Part model, mm, in its own coordinate system. A direction names the side the tool comes from. Round coordinates to 2 decimals unless told otherwise and drop trailing zeros. Write each loop counter-clockwise with the first axis right and the second up, starting at its lowest first coordinate (ties: lowest second). Pieces come first, ordered by that corner, then holes. Notation, with made-up numbers: M -37.5,41 L 12.5,41 A6 cw 12.5,51 Z; hole C 34.25,37.5 d3. An arc over 180 degrees is marked long. Use one line per item in the form item = value. Start each with the question number.
Item 1: Probe L1, parallel to Z at x = -18, y = 173; L2, parallel to Z at x = -14, y = 80.5; L3, parallel to Y at x = -21.5, z = 3.5. List the from-to ranges inside material, lowest first.
Item 2: Cut at B-B, the plane y = 94. Give the cut face in (x, z), then the cut area to 3 significant figures.
Item 3: Cut at A-A, the plane z = 3. Give the cut face in (x, y), then the cut area to 3 significant figures.
Item 4: Flat gauge pins, fed straight in: pin 1 Ø0.8 at (y, z) = (117.5, 6.5) entering from +X; pin 2 Ø3.5 at (x, z) = (-8.5, 2) entering from -Y; pin 3 Ø7.5 at (x, y) = (-4, 57) entering from +Z. Where does each tip first touch, or does it go through?
Item 5: Which spindle directions (+Z, -Z, +X, -X, +Y, -Y) get a long thin tool onto all of the face, cutting with end or side? Do faces 4 (the face through (-13, 89, 6)), 5 (the face through (-10, 89, 0)), 6 (the face through (-16.5, 174.58, 3.07)). Say none if no direction does.
Item 6: Mould opens along Z. For faces 1 (the face through (-22.9, 88.74, 3.55)), 2 (the face through (-19.5, -4.93, 2.93)), 3 (the face through (-15, 89, 3)) say: +Z half, -Z half, draft (parallel to the pull), parting line (faces both ways), or undercut.
Item 7: Cut at C-C, the plane x = -26.5. Give the cut face in (y, z).
Autodesk Fusion 360 part; units mm, degrees
sketch "Sketch1" plane through (0, 0, 0) normal (0, 1, 0) x (1, 0, 0)
  line L0 (-30, 0) -> (10, 0)
  line L1 (10, 0) -> (10, -1)
  line L2 (10, -1) -> (-15, -1)
  line L3 (-15, -1) -> (-15, -6)
  line L4 (-15, -6) -> (-10, -6)
  line L5 (-10, -6) -> (-10, -7)
  line L6 (-10, -7) -> (-16, -7)
  line L7 (-16, -7) -> (-30, 0)
  dimension "d1" = 40
  dimension "d2" = 1
sketch "Sketch2" plane through (0, 0, 0) normal (0, 1, 0) x (1, 0, 0)
extrude "Extrude1" add sketch "Sketch1" along normal blind 200
sketch "Sketch3" plane through (0, 0, 0) normal (0, -1, 0) x (1, 0, 0)
  line L0 (-10, 7) -> (-16, 7)
  line L1 (-16, 7) -> (-30, 0)
  line L2 (-30, 0) -> (10, 0)
  line L3 (10, 0) -> (10, 1)
  line L4 (10, 1) -> (-15, 1)
  line L5 (-15, 1) -> (-15, 6)
  line L6 (-15, 6) -> (-10, 6)
  line L7 (-10, 6) -> (-10, 7)
  circle A0 centre (-18, 3) radius 1.5
  dimension "d5" = 3
  dimension "d6" = 3
  dimension "d7" = 3
extrude "Extrude2" add sketch "Sketch3" along normal blind 10 contours A0
sketch "Sketch4" plane through (0, 0, 0) normal (0, 1, 0) x (1, 0, 0)
sketch "Sketch5" plane through (0, 200, 0) normal (0, 1, 0) x (-1, 0, 0)
  line L0 (16, 7) -> (10, 7)
  line L1 (10, 7) -> (10, 6)
  line L2 (10, 6) -> (15, 6)
  line L3 (15, 6) -> (15, 1)
  line L4 (15, 1) -> (-10, 1)
  line L5 (-10, 1) -> (-10, 0)
  line L6 (-10, 0) -> (30, 0)
  line L7 (30, 0) -> (16, 7)
  circle A0 centre (18, 3) radius 1.5
  dimension "d10" = 3
  dimension "d11" = 3
  dimension "d12" = 3
extrude "Extrude3" cut sketch "Sketch5" against normal blind 11 contours A0
sketch "Sketch6" plane through (0, 200, 0) normal (0, 1, 0) x (-1, 0, 0)
  line L0 (16, 7) -> (10, 7)
  line L1 (10, 7) -> (10, 6)
  line L2 (10, 6) -> (15, 6)
  line L3 (15, 6) -> (15, 1)
  line L4 (15, 1) -> (-10, 1)
  line L5 (-10, 1) -> (-10, 0)
  line L6 (-10, 0) -> (30, 0)
  line L7 (30, 0) -> (16, 7)
extrude "Extrude4" cut sketch "Sketch6" against normal blind 20
sketch "Sketch7" plane through (0, 0, 0) normal (0, 1, 0) x (1, 0, 0)
sketch "Sketch8" plane through (0, 180, 0) normal (0, 1, 0) x (-1, 0, 0)
  line L0 (30, 0) -> (16, 7)
  line L1 (16, 7) -> (10, 7)
  line L2 (10, 7) -> (10, 6)
  line L3 (10, 6) -> (15, 6)
  line L4 (15, 6) -> (15, 1)
  line L5 (15, 1) -> (-10, 1)
  line L6 (-10, 1) -> (-10, 0)
  line L7 (-10, 0) -> (30, 0)
  circle A0 centre (18, 3) radius 1.5
  dimension "d17" = 3
  dimension "d18" = 3
  dimension "d19" = 3
extrude "Extrude5" cut sketch "Sketch8" against normal blind 11 contours A0
Model answer:
q1.L1 = 0 to 1.5, 4.5 to 6
q1.L2 = 0 to 1, 6 to 7
q1.L3 = 0 to 180
q2.outline = M -30,0 L 10,0 L 10,1 L -15,1 L -15,6 L -10,6 L -10,7 L -16,7 Z
q2.area = 86.0 mm²
q3.outline = M -24,0 L -19.5,0 L -19.5,-10 L -16.5,-10 L -16.5,0 L -15,0 L -15,180 L -16.5,180 L -16.5,169 L -19.5,169 L -19.5,180 L -24,180 Z
q3.area = 1,620 mm²
q4.pin_1 = -10
q4.pin_2 = 0
q4.pin_3 = 1
q5.face_4 = +X, +Y, -Y
q5.face_5 = -Z, +X, -X, +Y, -Y
q5.face_6 = +Y
q6.face_1 = +Z half
q6.face_2 = parting line
q6.face_3 = undercut
q7.outline = M 0,0 L 180,0 L 180,1.75 L 0,1.75 Z
